from build123d import *

# Parameters (mm, degrees)
F2_R     = 7.8994
F3_DEPTH = 52.42406


with BuildPart() as f1:
    # F0 (on Right) → F1 (revolve)
    with BuildSketch(Plane.YZ):
        Polygon((0, 25.4), (0, 13.34897), (55.59806, 13.34897), (52.115666, 16.74876), (48.940666, 16.74876), (17.3736, 24.64943), (14.1986, 24.64943), (14.1986, 53.99913), (3.175, 53.99913), (3.175, 25.4), align=None)
    revolve(axis=Axis((0, -0.429692, 0), (0, 1, 0)))

    # F2 (on face) → F3 (cut, through all)
    with BuildSketch(Plane.XZ.offset(-3.175)):
        with Locations((0, 39.6494)):
            Circle(F2_R)
        with Locations((-39.6494, 0)):
            Circle(F2_R)
        with Locations((0, -39.6494)):
            Circle(F2_R)
        with Locations((39.6494, 0)):
            Circle(F2_R)
    extrude(amount=-F3_DEPTH, mode=Mode.SUBTRACT)


solid = f1.part
Can you work these out from the model? Positions are in its coordinate system, mm. A direction names the side the tool comes from. Coordinates: 2 decimals unless noted, no trailing zeros. Loops run counter-clockwise (first coordinate to the right, second up) from the corner with the lowest first, then second, coordinate; pieces in that order, holes last. Notation, with made-up numbers: (79.5, -27) - (99.5, -27) arc R17 cw to (99.5, -23) - close; hole circle Ø3 at (-19.75, 86). An arc over 180 degrees is marked (long way). Put each result on its own line as item: value. Start each with the question number.
Item 1: Suppose I cut it at B-B (z = 0). Please give me the cut outline in (x, y) (3 decimals).
Item 2: Suppose I cut it at C-C (x = -42.5). Please give me the cut outline in (y, z) (1 decimal).
Item 3: For pin 1 (20.5 mm diameter, centred on x = -39.65, z = 0, fed in from -Y) (3 decimals); pin 2 (6 mm diameter, centred on x = -30.5, z = 5, fed in from +Y); pin 3 (1.5 mm diameter, centred on x = -11, y = 25, fed in from +Z); pin 4 (1.5 mm diameter, centred on x = -4, z = 20.5, fed in from -Y), each with a flat end and sliding along its axis, tell me the tip position at first contact or that it passes through.
Item 4: If we mould it in two halves opening along X, with no side actions, what happens to faces 1 (the face through (-1.03, 8.61, 47.48)), 2 (the face through (-13.24, 55.38, -2.94)), 3 (the face through (1, 14.199, 25))? For each: +X half, -X half, draft (parallel to the pull), parting line (faces both ways), or undercut.
Item 5: Suppose I cut it at D-D (z = -46). Please give me the cut outline in (x, y) (3 decimals), and give its area (3 significant figures).
Item 6: If I drill on line 1 along X through (y, z) = (4, 7); line 2 along X through (y, z) = (16, 0); line 3 along Y through (x, z) = (31, -43) (3 decimals), over which ranges is the centre line in solid material (lowest first)?
Item 7: Suppose I cut it at A-A (x = 0). Please give me the cut outline in (y, z) (3 decimals).
Item 8: Which directions (+Z, -Z, +X, -X, +Y, -Y) give clear straight access to the entire face, cutting with the end or side of a thin tool? Please do faces 4 (the face through (-1.028, 8.61, -31.817)), 5 (the face through (-24.796, 1.565, -5.506)), 6 (the face through (20.784, 15.764, 13.251)).
Here are the results:
1. outline: (-53.999, 3.175) - (-47.549, 3.175) - (-47.549, 14.199) - (-53.999, 14.199) - close; (-31.75, 3.175) - (-25.4, 3.175) - (-25.4, 0) - (-13.349, 0) - (-13.349, 55.598) - (-16.749, 52.116) - (-16.749, 48.941) - (-24.649, 17.374) - (-24.649, 14.199) - (-31.75, 14.199) - close; (13.349, 0) - (25.4, 0) - (25.4, 3.175) - (31.75, 3.175) - (31.75, 14.199) - (24.649, 14.199) - (24.649, 17.374) - (16.749, 48.941) - (16.749, 52.116) - (13.349, 55.598) - close; (47.549, 3.175) - (53.999, 3.175) - (53.999, 14.199) - (47.549, 14.199) - close
2. outline: (3.2, -33.3) - (14.2, -33.3) - (14.2, -7.4) - (3.2, -7.4) - close; (3.2, 7.4) - (14.2, 7.4) - (14.2, 33.3) - (3.2, 33.3) - close
3. pin 1: y = 3.175
3. pin 2: y = 14.2
3. pin 3: z = 20.35
3. pin 4: y = 0
4. face 1: undercut
4. face 2: parting line
4. face 3: draft
5. outline: (-28.283, 3.175) - (-4.698, 3.175) - (-4.698, 14.199) - (-28.283, 14.199) - close; (4.698, 3.175) - (28.283, 3.175) - (28.283, 14.199) - (4.698, 14.199) - close
5. area: 520 mm²
6. line 1: -53.54 to -43.31, -35.99 to -11.37, 11.37 to 35.99, 43.31 to 53.54
6. line 2: -24.65 to -13.35, 13.35 to 24.65
6. line 3: 3.175 to 14.199
7. outline: (0, -25.4) - (3.175, -25.4) - (3.175, -31.75) - (14.199, -31.75) - (14.199, -24.649) - (17.374, -24.649) - (48.941, -16.749) - (52.116, -16.749) - (55.598, -13.349) - (0, -13.349) - close; (0, 13.349) - (55.598, 13.349) - (52.116, 16.749) - (48.941, 16.749) - (17.374, 24.649) - (14.199, 24.649) - (14.199, 31.75) - (3.175, 31.75) - (3.175, 25.4) - (0, 25.4) - close; (3.175, -53.999) - (14.199, -53.999) - (14.199, -47.549) - (3.175, -47.549) - close; (3.175, 47.549) - (14.199, 47.549) - (14.199, 53.999) - (3.175, 53.999) - close
8. face 4: +Y, -Y
8. face 5: -Y
8. face 6: +Y
